Verification items for the finished model (mm, model axes). Face numbers are marked on the shaded views. Give positions to 0.01 mm unless a question says otherwise; leave off trailing zeros. Order: outer loops, then holes, each group sorted by start corner. A loop starts at its lowest first (then second) coordinate and runs counter-clockwise, first axis right, second up. Notation, with made-up numbers: (16.5, 70.5) - (73.5, 70.5) arc R30 cw to (73.5, 105.5) - close; hole circle Ø9 at (10, 50.25). An arc over 180 degrees is marked (long way). Answer as a JSON object with one key per item and string values.
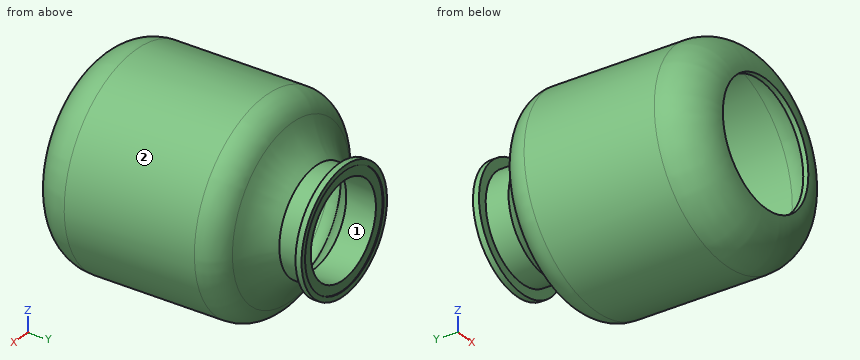
```python
from build123d import *


# Read off the part's stored shape, not the designer's step: Shell1
with BuildPart() as part:
    # Sketch1 → Revolve1 (revolve)
    with BuildSketch(Plane.XY, mode=Mode.PRIVATE) as revolve1_sk:
        with BuildLine():
            Line((0, 0), (24.360145845, 0))
            ThreePointArc((24.360145845, 0), (35.651483834, 4.677025332), (40.328509165, 15.96836332))
            Line((40.328509165, 15.96836332), (40.328509165, 67.23016629))
            ThreePointArc((40.328509165, 67.23016629), (38.415383352, 73.392914659), (33.348649325, 77.388878138))
            ThreePointArc((33.348649325, 77.388878138), (26.276782154, 81.308753559), (20.55607493, 87.022792188))
            Line((20.55607493, 87.022792188), (20.55607493, 96.024974169))
            Line((20.55607493, 96.024974169), (24.360145845, 96.024974169))
            Line((24.360145845, 96.024974169), (24.360145845, 98.393969428))
            Line((24.360145845, 98.393969428), (0, 98.393969428))
            Line((0, 98.393969428), (0, 0))
        make_face()
    revolve(revolve1_sk.sketch.rotate(Axis((0, 98.393969428, 0), (0, -1, 0)), 90), axis=Axis((0, 98.393969428, 0), (0, -1, 0)))

    # Shell1 outline → Shell1 (revolve, cut)
    with BuildSketch(Plane.XY):
        with BuildLine():
            Line((24.360145845, 0), (24.360145845, 2))
            ThreePointArc((24.360145845, 2), (34.237270271, 6.091238894), (38.328509165, 15.96836332))
            Line((38.328509165, 15.96836332), (38.328509165, 67.23016629))
            ThreePointArc((38.328509165, 67.23016629), (36.766977277, 72.260325849), (32.631406737, 75.521911864))
            ThreePointArc((32.631406737, 75.521911864), (24.803132334, 79.91715704), (18.55607493, 86.364973266))
            Line((18.55607493, 86.364973266), (18.55607493, 98.024974169))
            Line((18.55607493, 98.024974169), (22.360145845, 98.024974169))
            Line((22.360145845, 98.024974169), (22.360145845, 98.393969428))
            Line((22.360145845, 98.393969428), (0, 98.393969428))
            Line((0, 98.393969428), (0, 0))
            Line((0, 0), (24.360145845, 0))
        make_face()
    revolve(axis=Axis((0, 0, 0), (0, 1, 0)), mode=Mode.SUBTRACT)


solid = part.part
```
(1) Material ranges on line 1 along X through (y, z) = (28, 0); line 2 along X through (y, z) = (90, 0); line 3 along Y through (x, z) = (-34, -9), recorded low to high. Write a range as [from, to].
Computed values:
{"line 1": "x = [-40.33, -38.33], [38.33, 40.33]", "line 2": "x = [-20.56, -18.56], [18.56, 20.56]", "line 3": "y = [4.22, 7.12], [74.02, 76.49]"}
(2) Release check for a two-part mould opening along Z. For the marked faces 1 and 2 record: pulls with the +Z half, pulls with the -Z half, needs draft (parallel to the pull), parting line crosses it, or undercut.
Computed values:
{"face 1": "undercut", "face 2": "parting line crosses it"}
(3) Gauge pin test, flat ends, axial feed: pin 1 Ø12 at (x, y) = (27.5, 77.5) entering from +Z; pin 2 Ø6 at (x, z) = (12.5, -24.5) entering from -Y; pin 3 Ø22.5 at (x, z) = (-7, -7) entering from +Y (3 decimals). Record the tip position at first contact, or that the pin passes through.
Computed values:
{"pin 1": "stops at z = 30.7", "pin 2": "stops at y = 0", "pin 3": "stops at y = 98.025"}
(4) Section check C-C (y = 21.5). Record the cut outline in (x, z), then the cut area to 3 significant figures.
Computed values:
{"outline": "circle Ø80.66 at (0, 0); hole circle Ø76.66 at (0, 0)", "area": "494 mm²"}
(5) Section check D-D (y = 90). Record the cut outline in (x, z).
Computed values:
{"outline": "circle Ø41.11 at (0, 0); hole circle Ø37.11 at (0, 0)"}
